Check sheet for the drawn part. Datum: minimum x, y, z corner. Units: mm. Coordinates: 2 decimals unless noted, no trailing zeros. Write each loop counter-clockwise with the first axis right and the second up, starting at its lowest first coordinate (ties: lowest second). Pieces come first, ordered by that corner, then holes. Notation, with made-up numbers: (31, 86) -> (67, 86) arc R12 cw to (67, 108) -> close; hole circle Ø5 at (55, 73.5). An arc over 180 degrees is marked (long way). Answer in a Markdown table with one row per item. Add a question column.
Q1. Thickness scan on line 1 (Z direction, x = 5, y = 1.4); line 2 (X direction, y = 0.25, z = 3.25); line 3 (X direction, y = 0.75, z = 4). Record the ranges inside material, lowest first.
Q2. Section check B-B, the plane y = 0.4. Record the boundary of the cut face in (x, z).
Q3. Section check A-A, the plane x = 5. Record the boundary of the cut face in (y, z).
Q4. Section check C-C, the plane z = 8.25. Record the boundary of the cut face in (x, y), and give its area (3 significant figures).
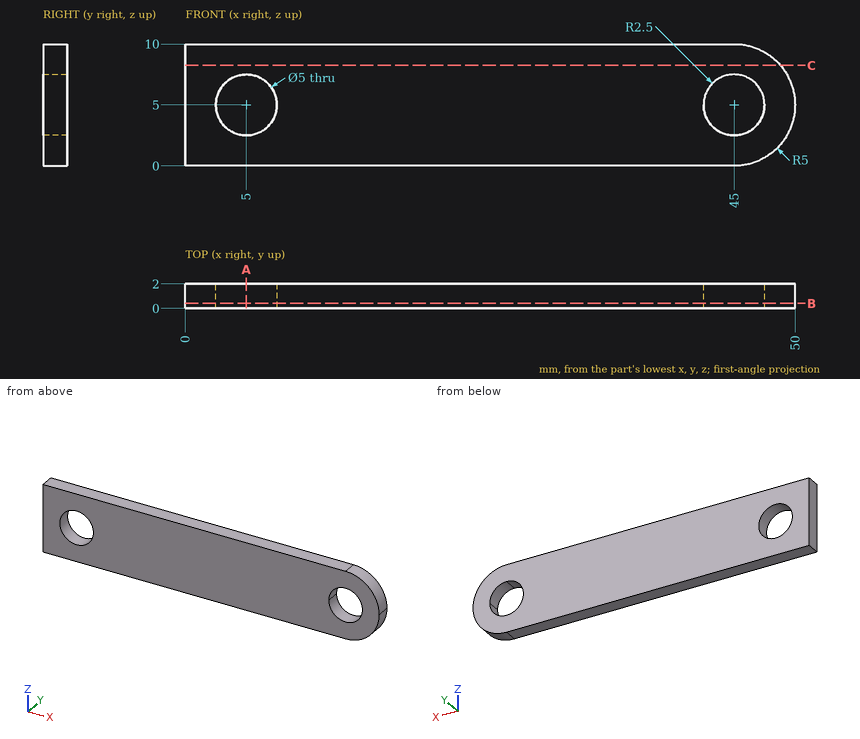
Calculated:
| question | item | result |
|---|---|---|
| 1 | line 1 | z = 0 to 2.5, 7.5 to 10 |
| 1 | line 2 | x = 0 to 3.21, 6.79 to 43.21, 46.79 to 49.68 |
| 1 | line 3 | x = 0 to 2.71, 7.29 to 42.71, 47.29 to 49.9 |
| 2 | outline | (0, 0) -> (45, 0) arc R5 ccw to (45, 10) -> (0, 10) -> close; hole circle Ø5 at (5, 5); hole circle Ø5 at (45, 5) |
| 3 | outline | (0, 0) -> (2, 0) -> (2, 2.5) -> (0, 2.5) -> close; (0, 7.5) -> (2, 7.5) -> (2, 10) -> (0, 10) -> close |
| 4 | outline | (0, 0) -> (48.8, 0) -> (48.8, 2) -> (0, 2) -> close |
| 4 | area | 97.6 mm² |
